CAD build for the part. Positions are in the model's coordinates, mm. A direction names the side the tool comes from. Round coordinates to 2 decimals unless told otherwise and drop trailing zeros. Loops run counter-clockwise (first coordinate to the right, second up) from the corner with the lowest first, then second, coordinate; pieces in that order, holes last. Notation, with made-up numbers: (79.5, 64) -> (87.5, 64) arc R33 ccw to (87.5, 99) -> close; hole circle Ø11 at (85, -27.75). An arc over 180 degrees is marked (long way). Answer as CSV lines item,"result".
Autodesk Inventor part; units mm, degrees
ref_plane "YZ Plane" through (0, 0, 0) normal (1, 0, 0) x (0, 1, 0)
ref_plane "XZ Plane" through (0, 0, 0) normal (0, 1, 0) x (-1, 0, 0)
ref_plane "XY Plane" through (0, 0, 0) normal (0, 0, 1) x (1, 0, 0)
sketch "Boceto1" plane through (0, 0, 0) normal (0, 0, 1) x (1, 0, 0)
  line L0 (-39.25, 25.5) -> (39.25, 25.5)
  line L1 (39.25, 25.5) -> (39.25, -25.5)
  line L2 (39.25, -25.5) -> (-39.25, -25.5)
  line L3 (-39.25, -25.5) -> (-39.25, 25.5)
  line L4 (-39.25, 25.5) -> (39.25, -25.5) construction
  line L5 (39.25, 25.5) -> (-39.25, -25.5) construction
  line L6 (42.25, 28.5) -> (-42.25, 28.5)
  line L7 (-42.25, 28.5) -> (-42.25, -28.5)
  line L8 (-42.25, -28.5) -> (42.25, -28.5)
  line L9 (42.25, -28.5) -> (42.25, 28.5)
  point P0 (0, 0)
  dimension "d0" = 51
  dimension "d1" = 78.5
  dimension "d2" = 3
extrude "Extrusión1" add sketch "Boceto1" along normal blind 4
sketch "Boceto2" plane through (0, 0, 0) normal (0, 0, -1) x (-1, 0, 0)
  line L0 (-42.25, 28.5) -> (42.25, 28.5)
  line L1 (42.25, -28.5) -> (-42.25, -28.5)
  line L2 (-42.25, 28.5) -> (42.25, 28.5)
  line L3 (42.25, 28.5) -> (42.25, -28.5)
  line L4 (42.25, -28.5) -> (-42.25, -28.5)
  line L5 (-42.25, -28.5) -> (-42.25, 28.5)
  point P0 (0, 0)
  point P1 (-42.25, -28.5)
extrude "Extrusión2" add sketch "Boceto2" along normal blind 15
sketch "Boceto3" plane through (0, 0, -15) normal (0, 0, -1) x (-1, 0, 0)
  line L0 (-33.5, 17.5) -> (33.5, 17.5)
  line L1 (33.5, 17.5) -> (33.5, -17.5)
  line L2 (33.5, -17.5) -> (-33.5, -17.5)
  line L3 (-33.5, -17.5) -> (-33.5, 17.5)
  line L4 (-33.5, 17.5) -> (33.5, -17.5) construction
  line L5 (33.5, 17.5) -> (-33.5, -17.5) construction
  line L6 (31.0225, -10) -> (35.9775, -10)
  line L7 (35.9775, -10) -> (35.9775, 10)
  line L8 (35.9775, 10) -> (31.0225, 10)
  line L9 (31.0225, 10) -> (31.0225, -10)
  line L10 (31.0225, -10) -> (35.9775, 10) construction
  line L11 (35.9775, -10) -> (31.0225, 10) construction
  line L12 (33.5, 10) -> (42.25, 10)
  line L13 (42.25, 28.5) -> (42.25, -28.5)
  line L14 (33.5, -10) -> (42.25, -10)
  line L15 (42.25, -10) -> (42.25, 10)
  line L16 (-20.5, 20.388) -> (-9.5, 20.388)
  line L17 (-9.5, 20.388) -> (-9.5, 14.612)
  line L18 (-9.5, 14.612) -> (-20.5, 14.612)
  line L19 (-20.5, 14.612) -> (-20.5, 20.388)
  line L20 (-20.5, 20.388) -> (-9.5, 14.612) construction
  line L21 (-9.5, 20.388) -> (-20.5, 14.612) construction
  line L22 (-42.25, 28.5) -> (42.25, 28.5)
  line L23 (-20.5, 17.5) -> (-9.5, 17.5)
  line L24 (-9.5, 17.5) -> (-9.5, 28.5)
  line L25 (-9.5, 28.5) -> (-20.5, 28.5)
  line L26 (-20.5, 28.5) -> (-20.5, 17.5)
  line L27 (-33.5, 0) -> (-37.4386, 0)
  line L28 (-20.5, -20.388) -> (-9.5, -20.388)
  line L29 (-9.5, -20.388) -> (-9.5, -14.612)
  line L30 (-9.5, -14.612) -> (-20.5, -14.612)
  line L31 (-20.5, -14.612) -> (-20.5, -20.388)
  line L32 (-20.5, -20.388) -> (-9.5, -14.612) construction
  line L33 (-9.5, -20.388) -> (-20.5, -14.612) construction
  line L34 (-20.5, -17.5) -> (-9.5, -17.5)
  line L35 (-9.5, -17.5) -> (-9.5, -28.5)
  line L36 (-9.5, -28.5) -> (-20.5, -28.5)
  line L37 (-20.5, -28.5) -> (-20.5, -17.5)
  point P0 (0, 0)
  point P1 (33.5, 0)
  point P2 (33.5, 10)
  point P3 (-15, 17.5)
  point P4 (-15, -17.5)
  point P5 (-20.5, -17.5)
  point P6 (-9.5, -17.5)
  point P7 (-20.5, 28.5)
  point P8 (-20.5, 17.5)
  point P9 (-9.5, 17.5)
  dimension "d7" = 67
  dimension "d8" = 35
  dimension "d9" = 20
  dimension "d33" = 11
  dimension "d34" = 13
  dimension "d38" = 0
extrude "Extrusión3" cut sketch "Boceto3" against normal blind 8 contours L0 L19 L18 L17 L1 L8 L9 L6 L2 L29 L30 L31 L3 | L19 L16 L17 L0 | L0 L17 L18 L19 | L26 L22 L24 L16 | L31 L30 L29 L2 | L2 L29 L28 L31 | L8 L7 L6 L1 | L1 L6 L9 L8 | L28 L35 L36 L37 | L12 L13 L14 L7
sketch "Boceto4" plane through (0, 0, 0) normal (0, 0, 1) x (1, 0, 0)
  line L0 (-42.05, -28.35) -> (-42.05, 28.35)
  line L1 (-42.05, 28.35) -> (42.05, 28.35)
  line L2 (42.05, 28.35) -> (42.05, -28.35)
  line L3 (42.05, -28.35) -> (-42.05, -28.35)
  line L4 (-42.05, -28.35) -> (42.05, 28.35) construction
  line L5 (-42.05, 28.35) -> (42.05, -28.35) construction
  line L6 (10.704, 28.35) -> (-32.296, 28.35)
  line L7 (42.05, 8.05) -> (42.05, 12.05)
  circle A0 centre (-37.05, -23.35) radius 2.25
  line L8 (-42.05, 12.05) -> (-42.05, -12.05)
  line L9 (-42.05, 0) -> (-48.6371, 0)
  line L10 (0, -28.35) -> (0, -35.954)
  circle A1 centre (-37.05, 23.35) radius 2.25
  circle A2 centre (37.05, -23.35) radius 2.25
  circle A3 centre (37.05, 23.35) radius 2.25
  point P0 (0, 0)
  point P1 (0, 0)
  dimension "d12" = 0
  dimension "d13" = 0
  dimension "d14" = 4.5
  dimension "d15" = 5
  dimension "d16" = 5
  dimension "d24" = 4.5
  dimension "d25" = 4.5
  dimension "d26" = 4.5
extrude "Extrusión4" cut sketch "Boceto4" against normal blind 15 contours A0 | A1 | A2 | A3
sketch "Boceto5" plane through (0, 0, 0) normal (0, 0, 1) x (1, 0, 0)
  circle A0 centre (-37.05, 23.35) radius 2.25
  line L0 (-39.25, 25.5) -> (39.25, 25.5)
  arc A1 (39.25, 23.8217) -> (37.7133, 25.5) centre (37.05, 23.35) ccw
  circle A2 centre (37.05, 23.35) radius 2.5
  circle A3 centre (37.05, -23.35) radius 2.25
  circle A4 centre (37.05, -23.35) radius 2.15
  line L1 (39.25, -25.5) -> (-39.25, -25.5)
  arc A5 (-36.3867, -25.5) -> (-39.25, -22.8783) centre (-37.05, -23.35) ccw
  circle A6 centre (-37.05, -23.35) radius 2.5
  circle A7 centre (-37.05, 23.35) radius 2.5
  circle A8 centre (37.05, -23.35) radius 2.5
  point P0 (0, 0)
  dimension "d28" = 5
  dimension "d29" = 4.5
  dimension "d30" = 5
  dimension "d31" = 5
  dimension "d32" = 5
extrude "Extrusión5" cut sketch "Boceto5" against normal blind 5 contours A2 L0 | L0 A2 | A4 | A6 L1 | L1 A6
sketch "Boceto6" plane through (-37.05, 23.35, -5) normal (0, 0, 1) x (1, 0, 0)
  circle A0 centre (0, 0) radius 4.2
  line L0 (37.05, 4.6715) -> (37.05, 10.9086)
  line L1 (-5.2, -13.35) -> (-5.2, -33.35)
  line L2 (-5.2, -23.35) -> (-13.3544, -23.35)
  circle A1 centre (74.1, 0) radius 4.2
  circle A2 centre (0, -46.7) radius 4.2
  circle A3 centre (74.1, -46.7) radius 4.2
  point P0 (37.05, -23.35)
  dimension "d21" = 8.4
extrude "Extrusión6" cut sketch "Boceto6" along normal blind 9
properties part number "bms_case"
Q1. Slice it at D-D, the plane y = 23.35. Give the cut face in (x, z), and give its area (3 significant figures).
Results:
outline,"(-42.25, -15) -> (-39.3, -15) -> (-39.3, -5) -> (-41.25, -5) -> (-41.25, 4) -> (-42.25, 4) -> close; (-34.8, -15) -> (9.5, -15) -> (9.5, -7) -> (20.5, -7) -> (20.5, -15) -> (34.8, -15) -> (34.8, -5) -> (32.85, -5) -> (32.85, 0) -> (-32.85, 0) -> (-32.85, -5) -> (-34.8, -5) -> close; (39.3, -15) -> (42.25, -15) -> (42.25, 4) -> (41.25, 4) -> (41.25, -5) -> (39.3, -5) -> close"
area,"1,010 mm2"
Q2. Tool access for faces 1 (the cylindrical face through (-40.146, -26.189, -1.563)), 2 (the flat face through (-33.5, 14, -11)), 3 (the flat face through (9.5, 23, -11)): list every direction of +Z, -Z, +X, -X, +Y, -Y with a clear straight run to the whole face (end or side of a thin tool).
Results:
face 1,"+Z"
face 2,"-Z"
face 3,"-Z, +Y, -Y"
Q3. Slice it at A-A, the plane x = -37.05. Give the cut face in (y, z).
Results:
outline,"(-28.5, -15) -> (-25.6, -15) -> (-25.6, -5) -> (-27.55, -5) -> (-27.55, 4) -> (-28.5, 4) -> close; (-21.1, -15) -> (-10, -15) -> (-10, -7) -> (10, -7) -> (10, -15) -> (21.1, -15) -> (21.1, -5) -> (19.15, -5) -> (19.15, 0) -> (-19.15, 0) -> (-19.15, -5) -> (-21.1, -5) -> close; (25.6, -15) -> (28.5, -15) -> (28.5, 4) -> (27.55, 4) -> (27.55, -5) -> (25.6, -5) -> close"
Q4. Slice it at C-C, the plane y = 12. Give the cut face in (x, z).
Results:
outline,"(-42.25, -15) -> (-33.5, -15) -> (-33.5, -7) -> (33.5, -7) -> (33.5, -15) -> (42.25, -15) -> (42.25, 4) -> (39.25, 4) -> (39.25, 0) -> (-39.25, 0) -> (-39.25, 4) -> (-42.25, 4) -> close"
Q5. Slice it at B-B, the plane z = -9.5. Give the cut face in (x, y).
Results:
outline,"(-42.25, -28.5) -> (9.5, -28.5) -> (9.5, -17.5) -> (-33.5, -17.5) -> (-33.5, -10) -> (-42.25, -10) -> close; (-42.25, 10) -> (-33.5, 10) -> (-33.5, 17.5) -> (9.5, 17.5) -> (9.5, 28.5) -> (-42.25, 28.5) -> close; (20.5, -28.5) -> (42.25, -28.5) -> (42.25, 28.5) -> (20.5, 28.5) -> (20.5, 17.5) -> (33.5, 17.5) -> (33.5, -17.5) -> (20.5, -17.5) -> close; hole circle Ø4.5 at (-37.05, -23.35); hole circle Ø4.5 at (-37.05, 23.35); hole circle Ø4.5 at (37.05, -23.35); hole circle Ø4.5 at (37.05, 23.35)"
Q6. Probe L1, parallel to Y at x = 37.05, z = -7.25; L2, parallel to X at y = -23.35, z = -2.5; L3, parallel to Y at x = -37.05, z = -1.75. List the from-to ranges inside material, lowest first. Write a range as [from, to].
Results:
L1,"[-28.5, -25.6], [-21.1, 21.1], [25.6, 28.5]"
L2,"[-42.25, -41.25], [-32.85, 32.85], [41.25, 42.25]"
L3,"[-28.5, -27.55], [-19.15, 19.15], [27.55, 28.5]"
Q7. Drop flat-ended pins along their axis: pin 1 Ø4 at (x, y) = (11, 10.5) entering from +Z; pin 2 Ø7.5 at (x, y) = (-37.05, -23.35) entering from +Z; pin 3 Ø4 at (x, y) = (-37.05, 23.35) entering from -Z; pin 4 Ø6 at (x, y) = (37.05, 23.35) entering from -Z. Give the stop position or say it passes through.
Results:
pin 1,"z = 0"
pin 2,"z = -5"
pin 3,"through"
pin 4,"z = -15"
Q8. Two-plate mould, pull along X, no slides. Class faces 4 (the cylindrical face through (39.31, -26.89, -1.56)), 5 (the flat face through (-38, 10, -11)), 6 (the cylindrical face through (36.76, 25.58, -9.93)), 7 (the flat face through (-42.25, 0, -6)): pulls with the +X half, pulls with the -X half, needs draft (parallel to the pull), parting line crosses it, or undercut.
Results:
face 4,"undercut"
face 5,"needs draft"
face 6,"undercut"
face 7,"pulls with the -X half"
